Model file for the job. Use its own axes, mm. A direction names the side the tool comes from. Give positions to 0.01 mm unless a question says otherwise; leave off trailing zeros. Loops run counter-clockwise (first coordinate to the right, second up) from the corner with the lowest first, then second, coordinate; pieces in that order, holes last. Notation, with made-up numbers: (32, 74.5) - (43, 74.5) arc R24 cw to (43, 100.5) - close; hole circle Ø3 at (-33, -33). An arc over 180 degrees is marked (long way). Use a Markdown table: item, result.
from build123d import *

# Parameters (mm, degrees)
F1_DEPTH  = 15.24
F2_DEPTH  = 12.7
F4_W      = 5.588
F4_H      = 3.048
F4_W_2    = 5.08
F4_H_2    = 2.481671654
F4_W_3    = 2.54
F4_H_3    = 2.6544967359
F5_DEPTH  = 6.604
F6_W      = 5.588
F6_H      = 3.048
F6_W_2    = 5.08
F6_H_2    = 2.481671654
F6_W_3    = 2.54
F6_H_3    = 2.6544967359
F7_DEPTH  = 6.604
F8_W      = 5.588
F8_H      = 3.048
F8_W_2    = 5.08
F8_H_2    = 2.481671654
F8_W_3    = 2.54
F8_H_3    = 2.6544967359
F9_DEPTH  = 6.604
F10_DEPTH = 3.175
F11_W     = 5.588
F11_H     = 3.048
F11_W_2   = 5.08
F11_H_2   = 2.481671654
F11_W_3   = 2.54
F11_H_3   = 2.6544967359
F12_DEPTH = 6.604
F14_DEPTH = 38.1


with BuildPart() as f1:
    # F0 (on Top) → F1 (new body)
    with BuildSketch(Plane.XY):
        Polygon((8.9802561211, 8.9802561211), (0, 17.9605122421), (-8.9802561211, 8.9802561211), (0, 0), align=None)
        Polygon((17.9605122421, 0), (8.9802561211, 8.9802561211), (0, 0), (8.9802561211, -8.9802561211), align=None)
        Polygon((0, 0), (-8.9802561211, -8.9802561211), (0, -17.9605122421), (8.9802561211, -8.9802561211), align=None)
        Polygon((-8.9802561211, 8.9802561211), (-17.9605122421, 0), (-8.9802561211, -8.9802561211), (0, 0), align=None)
    extrude(amount=F1_DEPTH)

    # F0 (on Top) → F2 (join)
    with BuildSketch(Plane.XY):
        Polygon((0, 17.9605122421), (-3.175, 17.9605122421), (-17.9605122421, 3.175), (-17.9605122421, 0), (-8.9802561211, 8.9802561211), align=None)
        Polygon((-8.9802561211, -8.9802561211), (-17.9605122421, 0), (-17.9605122421, -3.175), (-3.175, -17.9605122421), (0, -17.9605122421), align=None)
        Polygon((17.9605122421, -3.175), (17.9605122421, 0), (8.9802561211, -8.9802561211), (0, -17.9605122421), (3.175, -17.9605122421), align=None)
        Polygon((3.175, 17.9605122421), (0, 17.9605122421), (8.9802561211, 8.9802561211), (17.9605122421, 0), (17.9605122421, 3.175), align=None)
    extrude(amount=F2_DEPTH)

    # F4 (on face) → F5 (cut)
    with BuildSketch(Plane(origin=(-17.9605122421, 0, 0), x_dir=(0, -1, 0), z_dir=(-1, 0, 0))):
        with Locations((0, 10.824164173)):
            Rectangle(F4_W, F4_H)
        with Locations((0, 10.824164173)):
            Rectangle(F4_W_2, F4_H_2, mode=Mode.SUBTRACT)
        with Locations((0, 10.824164173)):
            Rectangle(F4_W_2, F4_H_2)
        with Locations((-1.27, 4.5022483679)):
            Rectangle(F4_W_3, F4_H_3)
        with Locations((1.27, 4.5022483679)):
            Rectangle(F4_W_3, F4_H_3)
        Polygon((0, 3.175), (-2.54, 3.175), (-2.54, 5.8294967359), (0, 5.8294967359), (0, 6.0262483679), (-2.794, 6.0262483679), (-2.794, 2.9782483679), (0, 2.9782483679), align=None)
        Polygon((2.54, 3.175), (0, 3.175), (0, 2.9782483679), (2.794, 2.9782483679), (2.794, 6.0262483679), (0, 6.0262483679), (0, 5.8294967359), (2.54, 5.8294967359), align=None)
    extrude(amount=-F5_DEPTH, mode=Mode.SUBTRACT)

    # F6 (on face) → F7 (cut)
    with BuildSketch(Plane.YZ.offset(17.9605122421)):
        with Locations((0, 10.824164173)):
            Rectangle(F6_W, F6_H)
        with Locations((0, 10.824164173)):
            Rectangle(F6_W_2, F6_H_2, mode=Mode.SUBTRACT)
        with Locations((0, 10.824164173)):
            Rectangle(F6_W_2, F6_H_2)
        with Locations((1.27, 4.5022483679)):
            Rectangle(F6_W_3, F6_H_3)
        with Locations((-1.27, 4.5022483679)):
            Rectangle(F6_W_3, F6_H_3)
        Polygon((0, 3.175), (-2.54, 3.175), (-2.54, 5.8294967359), (0, 5.8294967359), (0, 6.0262483679), (-2.794, 6.0262483679), (-2.794, 2.9782483679), (0, 2.9782483679), align=None)
        Polygon((2.54, 3.175), (0, 3.175), (0, 2.9782483679), (2.794, 2.9782483679), (2.794, 6.0262483679), (0, 6.0262483679), (0, 5.8294967359), (2.54, 5.8294967359), align=None)
    extrude(amount=-F7_DEPTH, mode=Mode.SUBTRACT)

    # F8 (on face) → F9 (cut)
    with BuildSketch(Plane.XZ.offset(17.9605122421)):
        with Locations((0, 10.824164173)):
            Rectangle(F8_W, F8_H)
        with Locations((0, 10.824164173)):
            Rectangle(F8_W_2, F8_H_2, mode=Mode.SUBTRACT)
        Polygon((2.54, 3.175), (0, 3.175), (0, 2.9782483679), (2.794, 2.9782483679), (2.794, 6.0262483679), (0, 6.0262483679), (0, 5.8294967359), (2.54, 5.8294967359), align=None)
        Polygon((0, 3.175), (-2.54, 3.175), (-2.54, 5.8294967359), (0, 5.8294967359), (0, 6.0262483679), (-2.794, 6.0262483679), (-2.794, 2.9782483679), (0, 2.9782483679), align=None)
        with Locations((-1.27, 4.5022483679)):
            Rectangle(F8_W_3, F8_H_3)
        with Locations((0, 10.824164173)):
            Rectangle(F8_W_2, F8_H_2)
        with Locations((1.27, 4.5022483679)):
            Rectangle(F8_W_3, F8_H_3)
    extrude(amount=-F9_DEPTH, mode=Mode.SUBTRACT)

    # F3 (on face) → F10 (join)
    with BuildSketch(Plane.XY.offset(12.7)):
        Polygon((0, 0), (8.9802561211, -8.9802561211), (13.4703841816, -4.4901280605), (0, 8.9802561211), (-2.2450640303, 6.7351920908), (2.2450640303, 2.2450640303), align=None)
        Polygon((4.4901280605, -13.4703841816), (8.9802561211, -8.9802561211), (0, 0), (-2.2450640303, -2.2450640303), (-6.7351920908, 2.2450640303), (-8.9802561211, 0), align=None)
    extrude(amount=F10_DEPTH)

    # F11 (on face) → F12 (cut)
    with BuildSketch(Plane(origin=(0, 17.9605122421, 0), x_dir=(-1, 0, 0), z_dir=(0, 1, 0))):
        Polygon((0, 3.175), (-2.54, 3.175), (-2.54, 5.8294967359), (0, 5.8294967359), (0, 6.0262483679), (-2.794, 6.0262483679), (-2.794, 2.9782483679), (0, 2.9782483679), align=None)
        Polygon((2.54, 3.175), (0, 3.175), (0, 2.9782483679), (2.794, 2.9782483679), (2.794, 6.0262483679), (0, 6.0262483679), (0, 5.8294967359), (2.54, 5.8294967359), align=None)
        with Locations((0, 10.824164173)):
            Rectangle(F11_W, F11_H)
        with Locations((0, 10.824164173)):
            Rectangle(F11_W_2, F11_H_2, mode=Mode.SUBTRACT)
        with Locations((-1.27, 4.5022483679)):
            Rectangle(F11_W_3, F11_H_3)
        with Locations((1.27, 4.5022483679)):
            Rectangle(F11_W_3, F11_H_3)
        with Locations((0, 10.824164173)):
            Rectangle(F11_W_2, F11_H_2)
    extrude(amount=-F12_DEPTH, mode=Mode.SUBTRACT)

    # F13 (on face) → F14 (cut)
    with BuildSketch(Plane(origin=(-10.5677561211, 10.5677561211, 0), x_dir=(-0.7071067812, -0.7071067812, 0), z_dir=(-0.7071067812, 0.7071067812, 0))):
        Polygon((-6.35, 2.38125), (0, 2.38125), (6.35, 2.38125), (6.35, 10.31875), (-6.35, 10.31875), align=None)
    extrude(amount=-F14_DEPTH, mode=Mode.SUBTRACT)


solid = f1.part
(1) Slice it at A-A, the plane z = 8. Write the cut outline in (x, y) (3 decimals).
Computed:
| item | result |
|---|---|
| outline | (-17.961, -3.175) - (-3.175, -17.961) - (3.175, -17.961) - (6.078, -15.058) - (-15.058, 6.078) - (-17.961, 3.175) - close; (-6.078, 15.058) - (15.058, -6.078) - (17.961, -3.175) - (17.961, 3.175) - (3.175, 17.961) - (-3.175, 17.961) - close |
(2) Pin check, flat tips, straight feed: P1, Ø1.7, axis at x = -16.5, y = 1, coming from the +Z side; P2, Ø5.5, axis at x = 11.5, y = 11.5, coming from the +Z side; P3, Ø1.5, axis at y = -0.5, z = 10.5, coming from the +X side; P4, Ø4.5, axis at x = -14, y = 1, coming from the -Z side. Stop position of each tip, or through.
Computed:
| item | result |
|---|---|
| P1 | z = 15.24 |
| P2 | z = 12.7 |
| P3 | x = 11.36 |
| P4 | z = 0 |
(3) Slice it at B-B, the plane z = 4.5. Count the separate pieces of the cut face and the enclosed holes in it, plus the area to 3 significant figures.
Computed:
| item | result |
|---|---|
| separate pieces | 6 |
| enclosed holes | 0 |
| area | 326 mm² |
(4) Drill centre lines: probe 1 along Z at (x, y) = (-9.5, 4); probe 2 along Z at (x, y) = (-7, -11); probe 3 along Z at (x, y) = (-1.5, -2) (3 decimals). Where is each one in solid material? Low to high. Write a range as [from, to].
Computed:
| item | result |
|---|---|
| probe 1 | [0, 2.38], [10.32, 15.24] |
| probe 2 | [0, 12.7] |
| probe 3 | [0, 2.381], [10.319, 15.875] |
(5) Slice it at C-C, the plane z = 10.75. Write the cut outline in (x, y) (3 decimals).
Computed:
| item | result |
|---|---|
| outline | (-17.961, -3.175) - (-3.175, -17.961) - (-2.794, -17.961) - (-2.794, -11.357) - (2.794, -11.357) - (2.794, -17.961) - (3.175, -17.961) - (17.961, -3.175) - (17.961, -2.794) - (11.357, -2.794) - (11.357, 2.794) - (17.961, 2.794) - (17.961, 3.175) - (3.175, 17.961) - (2.794, 17.961) - (2.794, 11.357) - (-2.794, 11.357) - (-2.794, 17.961) - (-3.175, 17.961) - (-17.961, 3.175) - (-17.961, 2.794) - (-11.357, 2.794) - (-11.357, -2.794) - (-17.961, -2.794) - close |
(6) Slice it at D-D, the plane x = -4. Write the cut outline in (y, z) (3 decimals), plus the area to 3 significant figures.
Computed:
| item | result |
|---|---|
| outline | (-17.136, 0) - (17.136, 0) - (17.136, 12.7) - (13.961, 12.7) - (13.961, 15.24) - (-0.49, 15.24) - (-0.49, 15.875) - (-4.98, 15.875) - (-4.98, 15.24) - (-13.961, 15.24) - (-13.961, 12.7) - (-17.136, 12.7) - close; hole (-4.98, 2.381) - (12.98, 2.381) - (12.98, 10.319) - (-4.98, 10.319) - close |
| area | 366 mm² |
(7) 3-axis set-ups, long thin cutter, end or side, ignore diameter. For faces 1 (the flat face through (-11.357, 0, 5)), 2 (the flat face through (0, 11.357, 11)), 3 (the flat face through (0, 1, 15.24)), 4 (the flat face through (-15, -2.794, 11)): which of +Z, -Z, +X, -X, +Y, -Y reach the whole face in a straight line?
Computed:
| item | result |
|---|---|
| face 1 | -X, +Y |
| face 2 | +Y |
| face 3 | +Z |
| face 4 | -X |
(8) Mould opens along X. For faces 5 (the flat face through (-2.34, -6.64, 15.55)), 6 (the flat face through (2.794, 15, 5)), 7 (the flat face through (0, 15, 6.026)), 8 (the flat face through (11.357, 0, 5)) say: pulls with the +X half, pulls with the -X half, needs draft (parallel to the pull), parting line crosses it, or undercut.
Computed:
| item | result |
|---|---|
| face 5 | pulls with the -X half |
| face 6 | undercut |
| face 7 | undercut |
| face 8 | pulls with the +X half |
